The listing builds one solid part. Answer for the finished solid, in the listing's coordinates (mm). A direction names the side the tool comes from. Round coordinates to 2 decimals unless told otherwise and drop trailing zeros. Answer in a Markdown table with one row per item.
from build123d import *

# Parameters (mm, degrees)
SKETCH1_R           = 9.525
ROUND_STOCK_DEPTH   = 3.175
SINGLE_TOOTH_DEPTH  = 15.892070037
TOOTH_PATTERN_COUNT = 13
CUT_EXTRUDE1_DEPTH  = 15.882187212
SKETCH8_R           = 3.81
BOSS_EXTRUDE1_DEPTH = 0.8382


with BuildPart() as part:
    # Sketch1 → Round Stock (new, symmetric)
    with BuildSketch(Plane.XY):
        Circle(SKETCH1_R)
    extrude(amount=ROUND_STOCK_DEPTH, both=True)

    # Sketch2 → Single Tooth (cut, through all)
    with BuildSketch(Plane.XY.offset(3.175)):
        with BuildLine():
            ThreePointArc((-8.699219347, -3.879330837), (-9.248220811, -2.279481702), (-9.505591122, -0.607751944))
            ThreePointArc((-9.505591122, -0.607751944), (-8.866874127, -0.859264513), (-8.194501154, -0.997585))
            ThreePointArc((-8.194501154, -0.997585), (-7.585039492, -1.044554082), (-6.973773022, -1.042846396))
            ThreePointArc((-6.973773022, -1.042846396), (-6.682727126, -1.135452938), (-6.520145475, -1.394008333))
            ThreePointArc((-6.520145475, -1.394008333), (-6.473754568, -1.595637192), (-6.421130074, -1.795729609))
            ThreePointArc((-6.421130074, -1.795729609), (-6.444932293, -2.100224502), (-6.659604229, -2.317479295))
            ThreePointArc((-6.659604229, -2.317479295), (-7.201647409, -2.600036906), (-7.71947129, -2.92485692))
            ThreePointArc((-7.71947129, -2.92485692), (-8.250547255, -3.35980093), (-8.699219347, -3.879330837))
        make_face()
    single_tooth = extrude(amount=-SINGLE_TOOTH_DEPTH, mode=Mode.SUBTRACT)

    # Tooth Pattern: Single Tooth ×13 about axis
    tooth_pattern_axis = Axis((0, 0, 0), (0, 0, 1))
    for i in range(1, TOOTH_PATTERN_COUNT):
        add(single_tooth.rotate(tooth_pattern_axis, i * 360 / TOOTH_PATTERN_COUNT), mode=Mode.SUBTRACT)

    # Sketch7 → Cut-Extrude1 (cut, through all)
    with BuildSketch(Plane(origin=(0, 0, -3.175), x_dir=(-1, 0, 0), z_dir=(0, 0, -1))):
        Polygon((1.3931462, -2.413), (2.786292399, 0), (1.3931462, 2.413), (-1.3931462, 2.413), (-2.786292399, 0), (-1.3931462, -2.413), align=None)
    extrude(amount=-CUT_EXTRUDE1_DEPTH, mode=Mode.SUBTRACT)

    # Sketch8 → Boss-Extrude1 (add)
    with BuildSketch(Plane.XY.offset(3.175)):
        Circle(SKETCH8_R)
        Polygon((-1.3931462, -2.413), (1.3931462, -2.413), (2.786292399, 0), (1.3931462, 2.413), (-1.3931462, 2.413), (-2.786292399, 0), align=None, mode=Mode.SUBTRACT)
    extrude(amount=BOSS_EXTRUDE1_DEPTH)


solid = part.part
(1) Flat-ended cylindrical pins translate along their axes: pin 1 (3 mm diameter, centred on y = -5.5, z = -0.5, fed in from +X); pin 2 (1 mm diameter, centred on x = -5.5, y = 3, fed in from +Z) (3 decimals); pin 3 (2 mm diameter, centred on x = -5.5, z = 1, fed in from +Y). Find the tip coordinate at first contact, or state that the pin passes through.
Checked values:
| item | result |
|---|---|
| pin 1 | stops at x = 7.52 |
| pin 2 | stops at z = 3.175 |
| pin 3 | stops at y = 8.17 |
(2) For faces 4 (the cylindrical face through (4.98, -5.81, 0.04)), 5 (the cylindrical face through (0.124, 7.647, 0.044)), 6 (the cylindrical face through (6.376, -4.254, 0.044)), 7 (the flat face through (0, -2.413, 0)), determine the directions among +Z, -Z, +X, -X, +Y, -Y from which every point of the face is accessible in a straight line to the end or side of a thin tool.
Checked values:
| item | result |
|---|---|
| face 4 | +Z, -Z, -Y |
| face 5 | +Z, -Z, +Y |
| face 6 | +Z, -Z, +X |
| face 7 | +Z, -Z |
(3) Find the intervals of material crossed by line 1 (Y direction, x = 7, z = 0); line 2 (X direction, y = -7, z = 0.25); line 3 (X direction, y = 7.25, z = -0.25), in increasing order.
Checked values:
| item | result |
|---|---|
| line 1 | y = -6.46 to -4.94, -2.8 to -0.65, 0.65 to 2.8, 4.94 to 6.46 |
| line 2 | x = -5.8 to -3.58, -1.91 to 0.2, 1.54 to 3.75 |
| line 3 | x = -5.86 to -3.78, -1.94 to 0.18, 1.63 to 3.82 |
(4) For a pull along X with two mould halves and no side action, classify faces 1 (the cylindrical face through (7.124, -6.323, 0.044)), 2 (the cylindrical face through (2.335, -8.588, 0.044)), 3 (the cylindrical face through (-8.43, 4.43, 0.04)) as pulls with the +X half, pulls with the -X half, needs draft (parallel to the pull), parting line crosses it, or undercut.
Checked values:
| item | result |
|---|---|
| face 1 | pulls with the +X half |
| face 2 | undercut |
| face 3 | pulls with the -X half |
